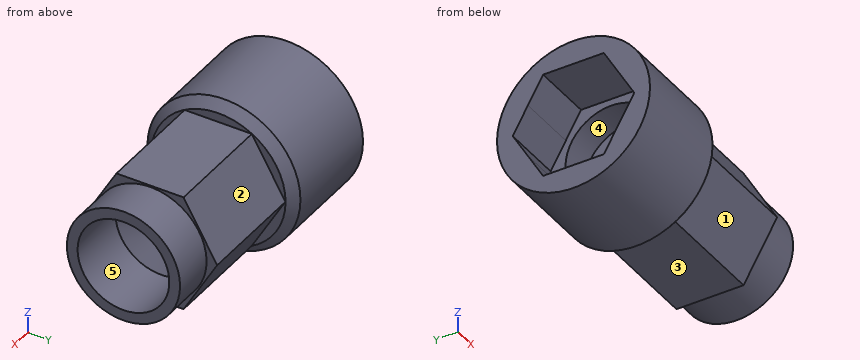
from build123d import *

# Parameters (mm, degrees)
F3_DEPTH  = 10
F5_DEPTH  = 18
F6_R      = 9.25
F7_DEPTH  = 7
F8_SIZE   = 1.5
F10_D     = 15
F10_DEPTH = 10
F10_TIP   = 4.5064546427


with BuildPart() as f1:
    # F0 (on Top) → F1 (revolve)
    with BuildSketch(Plane.XY):
        Polygon((0, 12.5), (0, 8.5), (10, 8.5), (10, 7.5), (15, 7.5), (15, 0), (18, 0), (18, 12.5), align=None)
    revolve(axis=Axis((16.5, 0, 0), (1, 0, 0)))

    # F2 (on face) → F3 (cut)
    with BuildSketch(Plane(origin=(0, 0, 0), x_dir=(0, -1, 0), z_dir=(-1, 0, 0))):
        with BuildLine():
            ThreePointArc((7.4478184814, -4.2999999846), (8.3069621084, -2.2258437793), (8.6, 0))
            ThreePointArc((8.6, 0), (8.3069621251, 2.2258437168), (7.4478185462, 4.2999998725))
            ThreePointArc((7.4478185462, 4.2999998725), (4.3000000638, 7.4478184357), (0, 8.6))
            ThreePointArc((0, 8.6), (-4.3000000291, 7.4478184557), (-7.4478185062, 4.2999999418))
            ThreePointArc((-7.4478185062, 4.2999999418), (-8.6, 4e-08), (-7.4478185462, -4.2999998725))
            ThreePointArc((-7.4478185462, -4.2999998725), (-4.3000000638, -7.4478184357), (0, -8.6))
            ThreePointArc((0, -8.6), (4.3000000077, -7.4478184681), (7.4478184814, -4.2999999846))
        make_face()
        with BuildLine():
            ThreePointArc((7.4478185462, 4.2999998725), (8.3069621251, 2.2258437168), (8.6, 0))
            ThreePointArc((8.6, 0), (8.3069621084, -2.2258437793), (7.4478184814, -4.2999999846))
            Line((7.4478184814, -4.2999999846), (9.9304246301, 0))
            Line((9.9304246301, 0), (7.4478185462, 4.2999998725))
        make_face()
        with BuildLine():
            ThreePointArc((0, 8.6), (4.3000000638, 7.4478184357), (7.4478185462, 4.2999998725))
            Line((7.4478185462, 4.2999998725), (4.965212315, 8.6))
            Line((4.965212315, 8.6), (0, 8.6))
        make_face()
        with BuildLine():
            Line((4.965212315, -8.6), (7.4478184814, -4.2999999846))
            ThreePointArc((7.4478184814, -4.2999999846), (4.3000000077, -7.4478184681), (0, -8.6))
            Line((0, -8.6), (4.965212315, -8.6))
        make_face()
        with BuildLine():
            ThreePointArc((-7.4478185062, 4.2999999418), (-4.3000000291, 7.4478184557), (0, 8.6))
            Line((0, 8.6), (-4.965212315, 8.6))
            Line((-4.965212315, 8.6), (-7.4478185062, 4.2999999418))
        make_face()
        with BuildLine():
            Line((-4.965212315, -8.6), (0, -8.6))
            ThreePointArc((0, -8.6), (-4.3000000638, -7.4478184357), (-7.4478185462, -4.2999998725))
            Line((-7.4478185462, -4.2999998725), (-4.965212315, -8.6))
        make_face()
        with BuildLine():
            ThreePointArc((-7.4478185462, -4.2999998725), (-8.6, 4e-08), (-7.4478185062, 4.2999999418))
            Line((-7.4478185062, 4.2999999418), (-9.9304246301, 0))
            Line((-9.9304246301, 0), (-7.4478185462, -4.2999998725))
        make_face()
    extrude(amount=-F3_DEPTH, mode=Mode.SUBTRACT)

    # F4 (on face) → F5 (join)
    with BuildSketch(Plane.YZ.offset(18)):
        Polygon((5.4848275573, 9.5), (-5.4848275573, 9.5), (-10.9696551146, 0), (-5.4848275573, -9.5), (5.4848275573, -9.5), (10.9696551146, 0), align=None)
    extrude(amount=F5_DEPTH)

    # F6 (on face) → F7 (join)
    with BuildSketch(Plane.YZ.offset(36)):
        Circle(F6_R)
    extrude(amount=F7_DEPTH)

    # F8
    f8_edges = [f1.edges().sort_by_distance(p)[0] for p in [
        (18, -12.5, 0),
    ]]
    chamfer(f8_edges, length=F8_SIZE)

    # F10
    with Locations(Plane.YZ.offset(43)):
        with Locations((0, 0)):
            Hole(F10_D / 2, depth=F10_DEPTH)
            with Locations((0, 0, -(F10_DEPTH + F10_TIP / 2))):  # 118° drill point
                Cone(0, F10_D / 2, F10_TIP, mode=Mode.SUBTRACT)


solid = f1.part
For this review, take the finished solid that the model builds, in its own axes (mm). Face numbers are marked on the shaded views. A direction names the side the tool comes from. Give positions to 0.01 mm unless a question says otherwise; leave off trailing zeros. Order: outer loops, then holes, each group sorted by start corner. A loop starts at its lowest first (then second) coordinate and runs counter-clockwise, first axis right, second up. Notation, with made-up numbers: (-18.75, 42) - (10.25, 42) arc R23 ccw to (10.25, 59) - close; hole circle Ø1 at (-19, 2). An arc over 180 degrees is marked (long way). Answer as a JSON object with one key per item and string values. Group by question number.
Item 1: Take a section at C-C on x = 37. Give the boundary of the cut face in (y, z).
Item 2: Clearance check with flat-ended pins moving along their axes: pin 1 Ø12 at (x, y) = (31.5, 2) entering from -Z; pin 2 Ø2 at (x, z) = (16.5, -9.5) entering from +Y; pin 3 Ø14 at (y, z) = (-1, 3) entering from -X; pin 4 Ø7.5 at (y, z) = (-2, -3) entering from -X. State where each tip first meets the part, or that it passes through.
Item 3: Take a section at A-A on x = 30. Give the boundary of the cut face in (y, z).
Item 4: Wall thickness on line 1 along Z through (x, y) = (37, 0); line 2 along Z through (x, y) = (13.3, 0); line 3 along X through (y, z) = (6, 8.5): over which ranges is each line inside the solid? List them lowest first.
Item 5: Take a section at B-B on x = 25. Give the boundary of the cut face in (y, z).
Item 6: Machinability: for the marked faces 1, 2, 3, 4 and 5, which of the approach directions +Z, -Z, +X, -X, +Y, -Y give a long, thin tool a straight path to every point of the face, cutting with its end or side? Answer none if there is none.
Reported:
{
 "1": {"outline": "circle Ø18.5 at (0, 0); hole circle Ø15 at (0, 0)"},
 "2": {"pin 1": "z = -9.5", "pin 2": "y = 9.17", "pin 3": "x = 0", "pin 4": "x = 15"},
 "3": {"outline": "(-10.97, 0) - (-5.48, -9.5) - (5.48, -9.5) - (10.97, 0) - (5.48, 9.5) - (-5.48, 9.5) - close; hole circle Ø5.01 at (0, 0)"},
 "4": {"line 1": "-9.25 to -7.5, 7.5 to 9.25", "line 2": "-12.5 to -7.5, 7.5 to 12.5", "line 3": "0 to 36"},
 "5": {"outline": "(-10.97, 0) - (-5.48, -9.5) - (5.48, -9.5) - (10.97, 0) - (5.48, 9.5) - (-5.48, 9.5) - close"},
 "6": {"face 1": "-Z, +X, -Y", "face 2": "+Z, +X, +Y", "face 3": "-Z, +X, +Y, -Y", "face 4": "-X", "face 5": "+X"}
}
